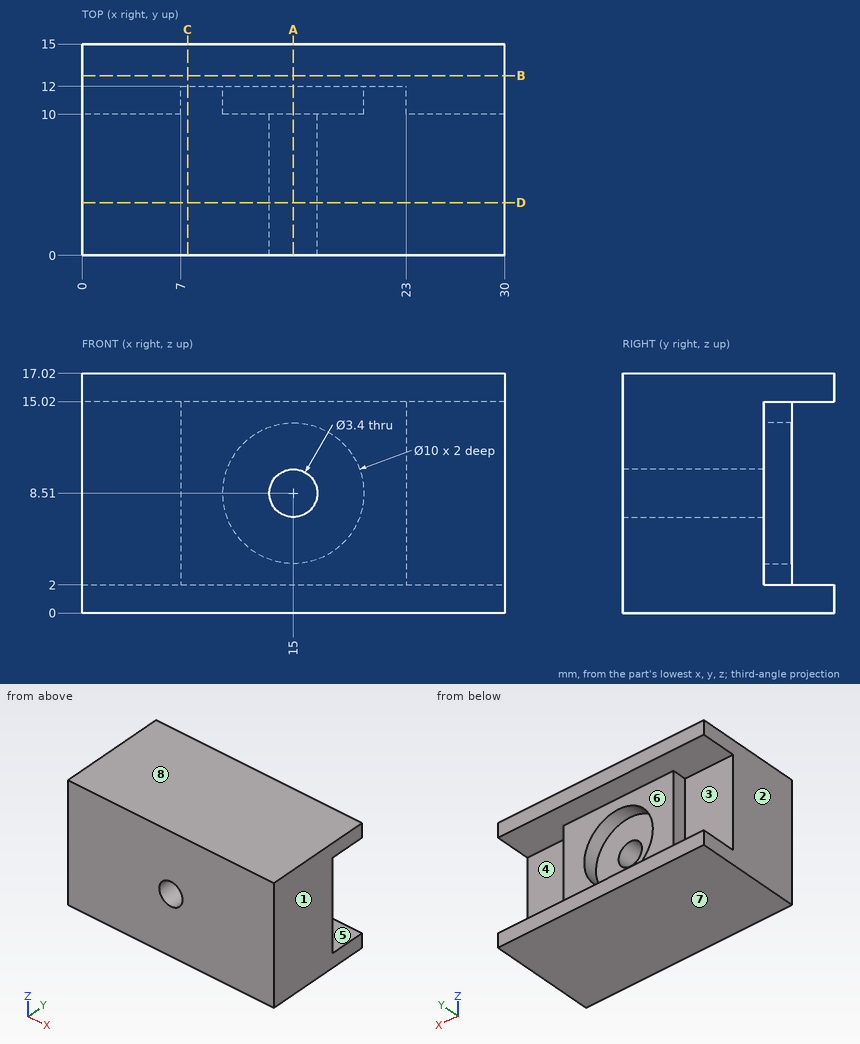
Drawing for the job (mm, zero at the part's lowest x, y, z). A direction names the side the tool comes from. Give positions to 0.01 mm unless a question says otherwise; leave off trailing zeros. Write each loop counter-clockwise with the first axis right and the second up, starting at its lowest first coordinate (ties: lowest second). Pieces come first, ordered by that corner, then holes. Notation, with made-up numbers: (45, 18) -> (84, 18) arc R19 ccw to (84, 54) -> close; hole circle Ø7 at (-20.75, 20.25). An arc over 180 degrees is marked (long way). Put each result on its own line as item: value. Start each with the question number.
Item 1: Cut at A-A (x = 15). List the corners of the cut face in (y, z).
Item 2: Cut at D-D (y = 3.75). List the corners of the cut face in (x, z), then the cut area to 3 significant figures.
Item 3: Cut at C-C (x = 7.5). List the corners of the cut face in (y, z).
Item 4: Wall check: L1, parallel to Z at x = 28.5, y = 11.75; L2, parallel to X at y = 11.5, z = 8.51; L3, parallel to X at y = 3.75, z = 8.51. Give the ranges that are in metal, low to high. Write a range as [from, to].
Item 5: Pull direction Z, two halves, no side cores. Call the marked faces 6, 7 and 8: pulls with the +Z half, pulls with the -Z half, needs draft (parallel to the pull), parting line crosses it, or undercut.
Item 6: Which spindle directions (+Z, -Z, +X, -X, +Y, -Y) get a long thin tool onto all of the face, cutting with end or side? Do the marked faces 1, 2, 3, 4 and 5. Say none if no direction does.
Item 7: Cut at B-B (y = 12.75). List the corners of the cut face in (x, z).
Item 8: Pin check, flat tips, straight feed: pin 1 Ø8 at (x, z) = (8, 10) entering from +Y; pin 2 Ø10 at (x, z) = (18, 3) entering from -Y; pin 3 Ø1.6 at (y, z) = (11.5, 5.5) entering from +X; pin 4 Ø3.5 at (x, z) = (2.5, 7) entering from +Y. Stop position of each tip, or through.
Answer list:
1. outline: (0, 0) -> (15, 0) -> (15, 2) -> (12, 2) -> (12, 3.51) -> (10, 3.51) -> (10, 6.81) -> (0, 6.81) -> close; (0, 10.21) -> (10, 10.21) -> (10, 13.51) -> (12, 13.51) -> (12, 15.02) -> (15, 15.02) -> (15, 17.02) -> (0, 17.02) -> close
2. outline: (0, 0) -> (30, 0) -> (30, 17.02) -> (0, 17.02) -> close; hole circle Ø3.4 at (15, 8.51)
2. area: 502 mm2
3. outline: (0, 0) -> (15, 0) -> (15, 2) -> (12, 2) -> (12, 15.02) -> (15, 15.02) -> (15, 17.02) -> (0, 17.02) -> close
4. L1: z = [0, 2], [15.02, 17.02]
4. L2: x = [7, 10], [20, 23]
4. L3: x = [0, 13.3], [16.7, 30]
5. face 6: undercut
5. face 7: pulls with the -Z half
5. face 8: pulls with the +Z half
6. face 1: +Z, -Z, +X, +Y, -Y
6. face 2: +Z, -Z, -X, +Y, -Y
6. face 3: -X, +Y
6. face 4: +X, +Y
6. face 5: +Y
7. outline: (0, 0) -> (30, 0) -> (30, 2) -> (0, 2) -> close; (0, 15.02) -> (30, 15.02) -> (30, 17.02) -> (0, 17.02) -> close
8. pin 1: stops at y = 12
8. pin 2: stops at y = 0
8. pin 3: stops at x = 23
8. pin 4: stops at y = 10
